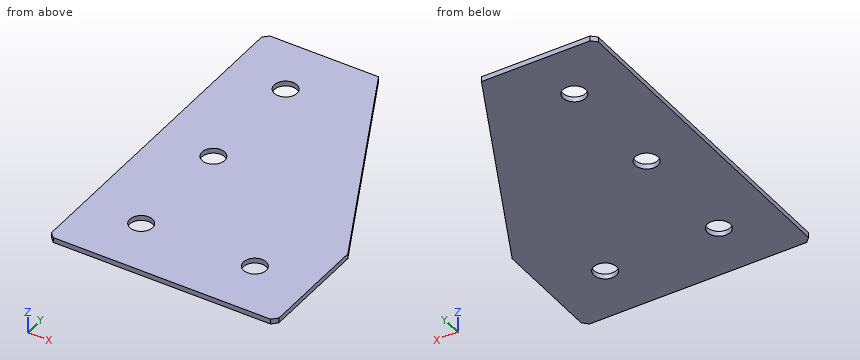
```python
from build123d import *

# Parameters (mm, degrees)
EXTRUDE_1_DEPTH   = 2
HOLE_WIZARD_M81_D = 9
CHAMFER_1_SIZE    = 2


with BuildPart() as part:
    # Эскиз1 → Бобышка-Вытянуть1 (new body)
    with BuildSketch(Plane(origin=(0, 0, 0), x_dir=(1, 0, 0), z_dir=(0, 0, -1))):
        Polygon((0, 0), (0, 135), (90, 135), (90, 90), (45, 0), align=None)
    extrude(amount=EXTRUDE_1_DEPTH)

    # Отверстие с зазором M81 (through all)
    with Locations(Plane(origin=(0, 0, -2), x_dir=(1, 0, 0), z_dir=(0, 0, -1))):
        with Locations((67.5, 112.5), (22.5, 112.5), (22.5, 67.5), (22.5, 22.5)):
            Hole(HOLE_WIZARD_M81_D / 2)

    # Фаска1
    chamfer_1_edges = [part.edges().sort_by_distance(p)[0] for p in [
        (0, 0, -1),
        (0, -135, -1),
        (90, -135, -1),
    ]]
    chamfer(chamfer_1_edges, length=CHAMFER_1_SIZE)


solid = part.part
```
CAD build for the part. Positions are in the model's coordinates, mm. Round coordinates to 2 decimals unless told otherwise and drop trailing zeros. Loops run counter-clockwise (first coordinate to the right, second up) from the corner with the lowest first, then second, coordinate; pieces in that order, holes last. Notation, with made-up numbers: M -22,41 L 22,41 A19 cw 22,50 Z; hole C 81.25,-15 d2. An arc over 180 degrees is marked long. Use a Markdown table: item, result. Add a question column.
(1) Cut at A-A (y = -67.5). Give the cut face in (x, z), and give its area (4 significant figures).
(2) Cut at B-B (x = 67.5). Give the cut face in (y, z), and give its area (3 significant figures).
(3) Cut at D-D (x = 22.5). Give the cut face in (y, z).
(4) Drill centre lines: line 1 (Y direction, x = 22.5, z = -0.8); line 2 (X direction, y = -112.5, z = -1.2); line 3 (X direction, y = -22.5, z = -0.8). Where is each one in solid material? Low to high.
(5) Cut at C-C (z = -0.75). Give the cut face in (x, y).
Geometry says:
| question | item | result |
|---|---|---|
| 1 | outline | M 0,-2 L 18,-2 L 18,0 L 0,0 Z; M 27,-2 L 78.75,-2 L 78.75,0 L 27,0 Z |
| 1 | area | 139.5 mm² |
| 2 | outline | M -135,-2 L -117,-2 L -117,0 L -135,0 Z; M -108,-2 L -45,-2 L -45,0 L -108,0 Z |
| 2 | area | 162 mm² |
| 3 | outline | M -135,-2 L -117,-2 L -117,0 L -135,0 Z; M -108,-2 L -72,-2 L -72,0 L -108,0 Z; M -63,-2 L -27,-2 L -27,0 L -63,0 Z; M -18,-2 L 0,-2 L 0,0 L -18,0 Z |
| 4 | line 1 | y = -135 to -117, -108 to -72, -63 to -27, -18 to 0 |
| 4 | line 2 | x = 0 to 18, 27 to 63, 72 to 90 |
| 4 | line 3 | x = 0 to 18, 27 to 56.25 |
| 5 | outline | M 0,-133 L 2,-135 L 88,-135 L 90,-133 L 90,-90 L 45,0 L 2,0 L 0,-2 Z; hole C 22.5,-112.5 d9; hole C 22.5,-67.5 d9; hole C 22.5,-22.5 d9; hole C 67.5,-112.5 d9 |
